Geometry check sheet. Reference: the model listing, model coordinates, mm. A direction names the side the tool comes from. Coordinates: 2 decimals unless noted, no trailing zeros. Write each loop counter-clockwise with the first axis right and the second up, starting at its lowest first coordinate (ties: lowest second). Pieces come first, ordered by that corner, then holes. Notation, with made-up numbers: M 24.25,53.25 L 72.25,53.25 A18 cw 72.25,82.25 Z; hole C -4,-37 d3. An arc over 180 degrees is marked long. Write each question's results on one line, items separated by ' | '.
```python
from build123d import *

# Parameters (mm, degrees)
EXTRUDE1_START       = -17
SKETCH1_W            = 42.3
SKETCH1_H            = 42.3
EXTRUDE1_DEPTH       = 9.6
CHAMFER3_SIZE        = 4
BOSS_EXTRUDE8_DEPTH  = 16.5
BOSS_EXTRUDE9_DEPTH  = 7.65
SKETCH33_R           = 11
BOSS_EXTRUDE10_DEPTH = 2
SKETCH34_R           = 5
CUT_EXTRUDE1_DEPTH   = 2
SKETCH35_R           = 2.5
BOSS_EXTRUDE11_DEPTH = 20
CUT_EXTRUDE3_DEPTH   = 15
SKETCH37_W           = 27.5
SKETCH37_H           = 16.5
BOSS_EXTRUDE12_DEPTH = 0.001
SKETCH38_W           = 27.5
SKETCH38_H           = 16.5
BOSS_EXTRUDE13_DEPTH = 0.001
SKETCH39_W           = 27.5
SKETCH39_H           = 16.5
BOSS_EXTRUDE14_DEPTH = 0.001
SKETCH40_W           = 27.5
SKETCH40_H           = 16.5
BOSS_EXTRUDE15_DEPTH = 0.001
SKETCH41_R           = 1.5
CUT_EXTRUDE4_DEPTH   = 6
SKETCH42_R           = 4.5
SKETCH42_R_2         = 1.5
CUT_EXTRUDE5_DEPTH   = 3
SKETCH43_W           = 16
SKETCH43_H           = 4
BOSS_EXTRUDE16_DEPTH = 3.2
SKETCH44_W           = 16
SKETCH44_H           = 6.4
BOSS_EXTRUDE17_DEPTH = 6
SKETCH45_W           = 15
SKETCH45_H           = 5.5
CUT_EXTRUDE6_DEPTH   = 5
SKETCH46_R           = 1.5
BOSS_EXTRUDE18_DEPTH = 1.5
CHAMFER4_SIZE        = 0.4


with BuildPart() as part:
    # Sketch1 → Extrude1 (new body)
    with BuildSketch(Plane(origin=(0, 0, 0), x_dir=(1, 0, 0), z_dir=(0, 1, 0)).offset(EXTRUDE1_START)):
        Rectangle(SKETCH1_W, SKETCH1_H)
    extrude(amount=EXTRUDE1_DEPTH)

    # Chamfer3
    chamfer3_edges = [part.edges().sort_by_distance(p)[0] for p in [
        (-21.15, -12.2, -21.15),
        (21.15, -12.2, -21.15),
        (21.15, -12.2, 21.15),
        (-21.15, -12.2, 21.15),
    ]]
    chamfer(chamfer3_edges, length=CHAMFER3_SIZE)

    # Sketch31 → Boss-Extrude8 (add)
    with BuildSketch(Plane(origin=(0, -7.4, 0), x_dir=(1, 0, 0), z_dir=(0, 1, 0))):
        Polygon((-13.75, 21.15), (13.75, 21.15), (21.15, 13.75), (21.15, -13.75), (13.75, -21.15), (-13.75, -21.15), (-21.15, -13.75), (-21.15, 13.75), align=None)
    extrude(amount=BOSS_EXTRUDE8_DEPTH)

    # Sketch32 → Boss-Extrude9 (add)
    with BuildSketch(Plane(origin=(0, 9.1, 0), x_dir=(1, 0, 0), z_dir=(0, 1, 0))):
        Polygon((-17.15, 21.15), (-21.15, 17.15), (-21.15, 13.75), (-21.15, -13.75), (-21.15, -17.15), (-17.15, -21.15), (-13.75, -21.15), (13.75, -21.15), (17.15, -21.15), (21.15, -17.15), (21.15, -13.75), (21.15, 13.75), (21.15, 17.15), (17.15, 21.15), (13.75, 21.15), (-13.75, 21.15), align=None)
    extrude(amount=BOSS_EXTRUDE9_DEPTH)

    # Sketch33 → Boss-Extrude10 (add)
    with BuildSketch(Plane(origin=(0, 16.75, 0), x_dir=(1, 0, 0), z_dir=(0, 1, 0))):
        Circle(SKETCH33_R)
    extrude(amount=BOSS_EXTRUDE10_DEPTH)

    # Sketch34 → Cut-Extrude1 (cut)
    with BuildSketch(Plane(origin=(0, 18.75, 0), x_dir=(1, 0, 0), z_dir=(0, 1, 0))):
        Circle(SKETCH34_R)
    extrude(amount=-CUT_EXTRUDE1_DEPTH, mode=Mode.SUBTRACT)

    # Sketch35 → Boss-Extrude11 (add)
    with BuildSketch(Plane(origin=(0, 16.75, 0), x_dir=(1, 0, 0), z_dir=(0, 1, 0))):
        Circle(SKETCH35_R)
    extrude(amount=BOSS_EXTRUDE11_DEPTH)

    # Sketch36 → Cut-Extrude3 (cut)
    with BuildSketch(Plane(origin=(0, 36.75, 0), x_dir=(1, 0, 0), z_dir=(0, 1, 0))):
        with BuildLine():
            Line((-1.275735082, 2.15), (0, 2.15))
            Line((0, 2.15), (1.275735082, 2.15))
            ThreePointArc((1.275735082, 2.15), (0, 2.5), (-1.275735082, 2.15))
        make_face()
    extrude(amount=-CUT_EXTRUDE3_DEPTH, mode=Mode.SUBTRACT)

    # Sketch37 → Boss-Extrude12 (add)
    with BuildSketch(Plane(origin=(21.15, 0, 0), x_dir=(0, 0, -1), z_dir=(1, 0, 0))):
        with Locations((0, 0.85)):
            Rectangle(SKETCH37_W, SKETCH37_H)
    extrude(amount=BOSS_EXTRUDE12_DEPTH)

    # Sketch38 → Boss-Extrude13 (add)
    with BuildSketch(Plane.XY.offset(21.15)):
        with Locations((0, 0.85)):
            Rectangle(SKETCH38_W, SKETCH38_H)
    extrude(amount=BOSS_EXTRUDE13_DEPTH)

    # Sketch39 → Boss-Extrude14 (add)
    with BuildSketch(Plane.ZY.offset(21.15)):
        with Locations((0, 0.85)):
            Rectangle(SKETCH39_W, SKETCH39_H)
    extrude(amount=BOSS_EXTRUDE14_DEPTH)

    # Sketch40 → Boss-Extrude15 (add)
    with BuildSketch(Plane(origin=(0, 0, -21.15), x_dir=(-1, 0, 0), z_dir=(0, 0, -1))):
        with Locations((0, 0.85)):
            Rectangle(SKETCH40_W, SKETCH40_H)
    extrude(amount=BOSS_EXTRUDE15_DEPTH)

    # Sketch41 → Cut-Extrude4 (cut)
    with BuildSketch(Plane(origin=(0, 16.75, 0), x_dir=(1, 0, 0), z_dir=(0, 1, 0))):
        with Locations((-15.5, 15.5)):
            Circle(SKETCH41_R)
        with Locations((-15.5, -15.5)):
            Circle(SKETCH41_R)
        with Locations((15.5, -15.5)):
            Circle(SKETCH41_R)
        with Locations((15.5, 15.5)):
            Circle(SKETCH41_R)
    extrude(amount=-CUT_EXTRUDE4_DEPTH, mode=Mode.SUBTRACT)

    # Sketch42 → Cut-Extrude5 (cut)
    with BuildSketch(Plane.XZ.offset(17)):
        Circle(SKETCH42_R)
        with Locations((-15.5, 15.5)):
            Circle(SKETCH42_R_2)
        with Locations((15.5, 15.5)):
            Circle(SKETCH42_R_2)
        with Locations((15.5, -15.5)):
            Circle(SKETCH42_R_2)
        with Locations((-15.5, -15.5)):
            Circle(SKETCH42_R_2)
    extrude(amount=-CUT_EXTRUDE5_DEPTH, mode=Mode.SUBTRACT)

    # Sketch43 → Boss-Extrude16 (add)
    with BuildSketch(Plane.XZ.offset(17)):
        with Locations((0, 23.15)):
            Rectangle(SKETCH43_W, SKETCH43_H)
    extrude(amount=-BOSS_EXTRUDE16_DEPTH)

    # Sketch44 → Boss-Extrude17 (add)
    with BuildSketch(Plane.XY.offset(21.15)):
        with Locations((0, -10.6)):
            Rectangle(SKETCH44_W, SKETCH44_H)
    extrude(amount=BOSS_EXTRUDE17_DEPTH)

    # Sketch45 → Cut-Extrude6 (cut)
    with BuildSketch(Plane.XY.offset(27.15)):
        with Locations((0, -10.65)):
            Rectangle(SKETCH45_W, SKETCH45_H)
    extrude(amount=-CUT_EXTRUDE6_DEPTH, mode=Mode.SUBTRACT)

    # Sketch46 → Boss-Extrude18 (add)
    with BuildSketch(Plane(origin=(0, 10.75, 0), x_dir=(1, 0, 0), z_dir=(0, 1, 0))):
        with Locations((-15.5, -15.5)):
            Circle(SKETCH46_R)
        with Locations((-15.5, 15.5)):
            Circle(SKETCH46_R)
        with Locations((15.5, 15.5)):
            Circle(SKETCH46_R)
        with Locations((15.5, -15.5)):
            Circle(SKETCH46_R)
    extrude(amount=BOSS_EXTRUDE18_DEPTH)

    # Chamfer4
    chamfer4_edges = [part.edges().sort_by_distance(p)[0] for p in [
        (-11, 18.75, 0),
    ]]
    chamfer(chamfer4_edges, length=CHAMFER4_SIZE)


solid = part.part
```
Q1. Sectioned sample at D-D on x = 18. Record the cut outline in (y, z), and give its area (3 significant figures).
Geometry check:
outline: M -17,-20.3 L -7.4,-20.3 L -7.4,-16.9 L 9.1,-16.9 L 9.1,-20.3 L 16.75,-20.3 L 16.75,20.3 L 9.1,20.3 L 9.1,16.9 L -7.4,16.9 L -7.4,20.3 L -17,20.3 Z | area: 1,260 mm2
Q2. Sectioned sample at B-B on x = -15.5. Record the cut outline in (y, z).
Geometry check:
outline: M -17,-21.15 L -7.4,-21.15 L -7.4,-19.4 L 9.1,-19.4 L 9.1,-21.15 L 16.75,-21.15 L 16.75,-17 L 12.25,-17 L 12.25,-14 L 16.75,-14 L 16.75,14 L 12.25,14 L 12.25,17 L 16.75,17 L 16.75,21.15 L 9.1,21.15 L 9.1,19.4 L -7.4,19.4 L -7.4,21.15 L -17,21.15 L -17,17 L -14,17 L -14,14 L -17,14 L -17,-14 L -14,-14 L -14,-17 L -17,-17 Z
Q3. Depth check by flat-ended pin: P1, Ø5, axis at x = -15.5, z = -15.5, coming from the -Y side; P2, Ø10, axis at x = -2, y = 13.5, coming from the +Z side; P3, Ø3.5, axis at x = 15.5, z = 15.5, coming from the +Y side; P4, Ø1.8, axis at y = -13, z = 23.5, coming from the -X side. Enter the tip coordinate at first touch or a pass-through.
Geometry check:
P1: stops at y = -17 | P2: stops at z = 21.15 | P3: stops at y = 16.75 | P4: stops at x = -8
Q4. Access from +Z, -Z, +X, -X, +Y, -Y to the whole of each face (thin tool, end or side, straight path). Record for faces 4 (the flat face through (0, -7.9, 25)), 5 (the flat face through (-18, 9.1, 18)), 6 (the cylindrical face through (14, -15.52, 15.57)).
Geometry check:
face 4: +Z | face 5: +Z, -X | face 6: -Y
Q5. Sectioned sample at A-A on y = 15.5. Record the cut outline in (x, z).
Geometry check:
outline: M -21.15,-17.15 L -17.15,-21.15 L 17.15,-21.15 L 21.15,-17.15 L 21.15,17.15 L 17.15,21.15 L -17.15,21.15 L -21.15,17.15 Z; hole C -15.5,-15.5 d3; hole C -15.5,15.5 d3; hole C 15.5,-15.5 d3; hole C 15.5,15.5 d3
Q6. Scan lines: probe 1 along Z at (x, y) = (-15.5, -15.95); probe 2 along Z at (x, y) = (0, -16); probe 3 along Z at (x, y) = (-12.5, -13.5). Record each from-to range of solid material in increasing order.
Geometry check:
probe 1: z = -21.15 to -17, -14 to 14, 17 to 21.15 | probe 2: z = -21.15 to -4.5, 4.5 to 25.15 | probe 3: z = -21.15 to 21.15
Q7. Mould release check, pull along Y, two halves, no side actions. Record for faces 1 (the flat face through (7.5, -11, 25)), 2 (the flat face through (5, 18.75, 2)), 3 (the flat face through (0, 1, 21.151)): pulls with the +Y half, pulls with the -Y half, needs draft (parallel to the pull), parting line crosses it, or undercut.
Geometry check:
face 1: undercut | face 2: pulls with the +Y half | face 3: needs draft
